```python
from build123d import *

# Parameters (mm, degrees)
F0_R     = 1.65
F1_DEPTH = 3


with BuildPart() as f1:
    # F0 (on Top) → F1 (new body)
    with BuildSketch(Plane.XY):
        with BuildLine():
            ThreePointArc((-24.535898, 34.063666), (-27.535898, 33.259818), (-29.732051, 31.063666))
            Line((-29.732051, 31.063666), (-41.767949, 10.216878))
            ThreePointArc((-41.767949, 10.216878), (-42.571797, 7.216878), (-41.767949, 4.216878))
            Line((-41.767949, 4.216878), (-17.232051, -38.280544))
            ThreePointArc((-17.232051, -38.280544), (-15.035898, -40.476697), (-12.035898, -41.280544))
            Line((-12.035898, -41.280544), (12.035898, -41.280544))
            ThreePointArc((12.035898, -41.280544), (15.035898, -40.476697), (17.232051, -38.280544))
            Line((17.232051, -38.280544), (41.767949, 4.216878))
            ThreePointArc((41.767949, 4.216878), (42.571797, 7.216878), (41.767949, 10.216878))
            Line((41.767949, 10.216878), (29.732051, 31.063666))
            ThreePointArc((29.732051, 31.063666), (27.535898, 33.259818), (24.535898, 34.063666))
            Line((24.535898, 34.063666), (-24.535898, 34.063666))
        make_face()
        with Locations((-12.5, -36.084392)):
            Circle(F0_R, mode=Mode.SUBTRACT)
        with Locations((0, -36.290163)):
            Circle(F0_R, mode=Mode.SUBTRACT)
        with Locations((12.5, -36.084392)):
            Circle(F0_R, mode=Mode.SUBTRACT)
        with BuildLine():
            Line((6.267949, -28.290163), (-6.267949, -28.290163))
            ThreePointArc((-6.267949, -28.290163), (-7.767949, -27.888239), (-8.866025, -26.790163))
            Line((-8.866025, -26.790163), (-27.633975, 5.716878))
            ThreePointArc((-27.633975, 5.716878), (-28.035898, 7.216878), (-27.633975, 8.716878))
            Line((-27.633975, 8.716878), (-21.366025, 19.573285))
            ThreePointArc((-21.366025, 19.573285), (-20.267949, 20.671361), (-18.767949, 21.073285))
            Line((-18.767949, 21.073285), (18.767949, 21.073285))
            ThreePointArc((18.767949, 21.073285), (20.267949, 20.671361), (21.366025, 19.573285))
            Line((21.366025, 19.573285), (27.633975, 8.716878))
            ThreePointArc((27.633975, 8.716878), (28.035898, 7.216878), (27.633975, 5.716878))
            Line((27.633975, 5.716878), (8.866025, -26.790163))
            ThreePointArc((8.866025, -26.790163), (7.767949, -27.888239), (6.267949, -28.290163))
        make_face(mode=Mode.SUBTRACT)
        with Locations((-37.5, 7.216878)):
            Circle(F0_R, mode=Mode.SUBTRACT)
        with Locations((-25, 28.867513)):
            Circle(F0_R, mode=Mode.SUBTRACT)
        with Locations((37.5, 7.216878)):
            Circle(F0_R, mode=Mode.SUBTRACT)
        with Locations((25, 28.867513)):
            Circle(F0_R, mode=Mode.SUBTRACT)
    extrude(amount=F1_DEPTH)


solid = f1.part
```
The model under review builds one solid part; all positions refer to its coordinate system, in mm. A direction names the side the tool comes from. Round coordinates to 2 decimals unless told otherwise and drop trailing zeros. Order: outer loops, then holes, each group sorted by start corner. A loop starts at its lowest first (then second) coordinate and runs counter-clockwise, first axis right, second up.
(1) Take a section at B-B, the plane z = 0.55. Count the separate pieces of the cut face and the enclosed holes in it, plus the area to 3 significant figures.
Working result:
separate pieces: 1
enclosed holes: 8
area: 2,740 mm2
(2) Tool access review of faces 4 (the face through (18.38, -10.31, 1.48)), 5 (the face through (35.834, 20.494, 1.479)): name each direction out of +Z, -Z, +X, -X, +Y, -Y from which nothing blocks a thin tool from reaching the whole face with its end or side.
Working result:
face 4: +Z, -Z
face 5: +Z, -Z, +X, +Y
(3) Take a section at D-D, the plane y = 2.5. State the section outline as (x, z) points, plus the area to 3 significant figures.
Working result:
outline: (-40.78, 0) - (-25.78, 0) - (-25.78, 3) - (-40.78, 3) - close; (25.78, 0) - (40.78, 0) - (40.78, 3) - (25.78, 3) - close
area: 90.0 mm2
(4) Take a section at C-C, the plane x = 37.5. State the section outline as (y, z) points, plus the area to 3 significant figures.
Working result:
outline: (-3.18, 0) - (5.57, 0) - (5.57, 3) - (-3.18, 3) - close; (8.87, 0) - (17.61, 0) - (17.61, 3) - (8.87, 3) - close
area: 52.5 mm2
(5) Take a section at A-A, the plane x = 0. State the section outline as (y, z) points.
Working result:
outline: (-41.28, 0) - (-37.94, 0) - (-37.94, 3) - (-41.28, 3) - close; (-34.64, 0) - (-28.29, 0) - (-28.29, 3) - (-34.64, 3) - close; (21.07, 0) - (34.06, 0) - (34.06, 3) - (21.07, 3) - close
(6) Wall thickness on L1, parallel to Y at x = 0, z = 1.4; L2, parallel to X at y = 7, z = 0.2; L3, parallel to Y at x = -11, z = 0.5: over which ranges is each line inside the solid? List them lowest first.
Working result:
L1: y = -41.28 to -37.94, -34.64 to -28.29, 21.07 to 34.06
L2: x = -42.57 to -39.14, -35.86 to -28.03, 28.03 to 35.86, 39.14 to 42.57
L3: y = -41.28 to -36.77, -35.4 to -23.09, 21.07 to 34.06
(7) Mouldability with a two-part tool opening along Y and no side actions: class faces 1 (the face through (42.57, 7.17, 1.48)), 2 (the face through (-29.672, -16.734, 1.479)), 3 (the face through (0.761, -37.754, 1.479)) as released by +Y, released by -Y, zero draft, split by the parting line, or undercut.
Working result:
face 1: split by the parting line
face 2: released by -Y
face 3: undercut
